```python
from build123d import *

# Parameters (mm, degrees)
SKETCH1_W           = 130
SKETCH1_H           = 79
BOSS_EXTRUDE1_DEPTH = 30
FILLET1_R           = 6
SHELL1_T            = -2.5
SKETCH2_W           = 130
SKETCH2_H           = 79
SKETCH2_W_2         = 127.5
SKETCH2_H_2         = 76.5
CUT_EXTRUDE1_DEPTH  = 3
SKETCH3_R           = 2
BOSS_EXTRUDE2_DEPTH = 8
BOSS_EXTRUDE3_REACH = 83.763
CUT_EXTRUDE2_REACH  = 108.611
SKETCH5_W           = 31.98
SKETCH5_H           = 7.98
SKETCH6_W           = 41.4
SKETCH6_H           = 24.3
CUT_EXTRUDE3_DEPTH  = 1.25
CUT_EXTRUDE4_REACH  = 108.611
SKETCH7_R           = 3.26


with BuildPart() as part:
    # Sketch1 → Boss-Extrude1 (new body)
    with BuildSketch(Plane(origin=(0, 0, 0), x_dir=(1, 0, 0), z_dir=(0, 1, 0))):
        Rectangle(SKETCH1_W, SKETCH1_H)
    extrude(amount=BOSS_EXTRUDE1_DEPTH)

    # Fillet1
    fillet1_edges = [part.edges().sort_by_distance(p)[0] for p in [
        (0, 0, 39.5),
        (-65, 0, 0),
        (0, 0, -39.5),
        (65, 0, 0),
    ]]
    fillet(fillet1_edges, radius=FILLET1_R)

    # Shell1
    shell1_openings = [part.faces().sort_by_distance(p)[0] for p in [
        (0, 30, 0),
    ]]
    offset(amount=SHELL1_T, openings=shell1_openings)

    # Sketch2 → Cut-Extrude1 (cut)
    with BuildSketch(Plane(origin=(0, 30, 0), x_dir=(1, 0, 0), z_dir=(0, 1, 0))):
        Rectangle(SKETCH2_W, SKETCH2_H)
        Rectangle(SKETCH2_W_2, SKETCH2_H_2, mode=Mode.SUBTRACT)
    extrude(amount=-CUT_EXTRUDE1_DEPTH, mode=Mode.SUBTRACT)

    # Sketch3 → Boss-Extrude2 (add)
    with BuildSketch(Plane(origin=(0, 2.5, 0), x_dir=(1, 0, 0), z_dir=(0, 1, 0))):
        with Locations(Location((-47.503765377, 21.122596556, 0), (0, 0, 90))):
            Circle(SKETCH3_R)
        with Locations(Location((33.776234623, 21.122596556, 0), (0, 0, 90))):
            Circle(SKETCH3_R)
        with Locations(Location((-47.503765377, -13.167403444, 0), (0, 0, 90))):
            Circle(SKETCH3_R)
        with Locations(Location((33.776234623, -13.167403444, 0), (0, 0, 90))):
            Circle(SKETCH3_R)
    extrude(amount=BOSS_EXTRUDE2_DEPTH)

    # Sketch4 → Boss-Extrude3 (add, up to next)
    with BuildSketch(Plane(origin=(0, 30, 0), x_dir=(1, 0, 0), z_dir=(0, 1, 0)), mode=Mode.PRIVATE) as boss_extrude3_sk1:
        with BuildLine():
            Line((-62.5, 37), (-62.5, 35.502936105))
            ThreePointArc((-62.5, 35.502936105), (-58.382233047, 32.882233047), (-61.002936105, 37))
            Line((-61.002936105, 37), (-62.5, 37))
        make_face()
    boss_extrude3_tool1 = extrude(boss_extrude3_sk1.sketch, amount=-BOSS_EXTRUDE3_REACH, mode=Mode.PRIVATE) - part.part
    # Sketch4 → Boss-Extrude3 (add, up to next)
    with BuildSketch(Plane(origin=(0, 30, 0), x_dir=(1, 0, 0), z_dir=(0, 1, 0)), mode=Mode.PRIVATE) as boss_extrude3_sk2:
        with BuildLine():
            Line((62.5, 37), (62.5, 35.502936105))
            ThreePointArc((62.5, 35.502936105), (58.382233047, 32.882233047), (61.002936105, 37))
            Line((61.002936105, 37), (62.5, 37))
        make_face()
    boss_extrude3_tool2 = extrude(boss_extrude3_sk2.sketch, amount=-BOSS_EXTRUDE3_REACH, mode=Mode.PRIVATE) - part.part
    # Sketch4 → Boss-Extrude3 (add, up to next)
    with BuildSketch(Plane(origin=(0, 30, 0), x_dir=(1, 0, 0), z_dir=(0, 1, 0)), mode=Mode.PRIVATE) as boss_extrude3_sk3:
        with BuildLine():
            Line((-62.5, -37), (-62.5, -35.502936105))
            ThreePointArc((-62.5, -35.502936105), (-58.382233047, -32.882233047), (-61.002936105, -37))
            Line((-61.002936105, -37), (-62.5, -37))
        make_face()
    boss_extrude3_tool3 = extrude(boss_extrude3_sk3.sketch, amount=-BOSS_EXTRUDE3_REACH, mode=Mode.PRIVATE) - part.part
    # Sketch4 → Boss-Extrude3 (add, up to next)
    with BuildSketch(Plane(origin=(0, 30, 0), x_dir=(1, 0, 0), z_dir=(0, 1, 0)), mode=Mode.PRIVATE) as boss_extrude3_sk4:
        with BuildLine():
            Line((62.5, -37), (61.002936105, -37))
            ThreePointArc((61.002936105, -37), (58.382233047, -32.882233047), (62.5, -35.502936105))
            Line((62.5, -35.502936105), (62.5, -37))
        make_face()
    boss_extrude3_tool4 = extrude(boss_extrude3_sk4.sketch, amount=-BOSS_EXTRUDE3_REACH, mode=Mode.PRIVATE) - part.part
    add(boss_extrude3_tool1.solids().sort_by_distance((-60.224191, 30, -34.724191))[0])
    add(boss_extrude3_tool2.solids().sort_by_distance((60.224191, 30, -34.724191))[0])
    add(boss_extrude3_tool3.solids().sort_by_distance((-60.224191, 30, 34.724191))[0])
    add(boss_extrude3_tool4.solids().sort_by_distance((60.224191, 30, 34.724191))[0])

    # Cut-Extrude2: up to this face of the body (flat: up to its plane)
    cut_extrude2_end = Plane(part.part.faces().sort_by_distance((0, 18, 37))[0])
    # Sketch5 → Cut-Extrude2 (cut, up to the picked face)
    with BuildSketch(Plane.XY.offset(39.5), mode=Mode.PRIVATE) as cut_extrude2_sk1:
        with Locations((0, 26.01)):
            Rectangle(SKETCH5_W, SKETCH5_H)
    cut_extrude2_tool1 = split(extrude(cut_extrude2_sk1.sketch, amount=-CUT_EXTRUDE2_REACH, mode=Mode.PRIVATE), bisect_by=cut_extrude2_end, keep=Keep.BOTH, mode=Mode.PRIVATE)
    add(cut_extrude2_tool1.solids().sort_by(Axis((0, 26.01, 39.5), (0, 0, -1)))[0], mode=Mode.SUBTRACT)

    # Sketch6 → Cut-Extrude3 (cut)
    with BuildSketch(Plane(origin=(0, 0, 37), x_dir=(-1, 0, 0), z_dir=(0, 0, -1))):
        with Locations((0, 22.66)):
            Rectangle(SKETCH6_W, SKETCH6_H)
    extrude(amount=-CUT_EXTRUDE3_DEPTH, mode=Mode.SUBTRACT)

    # Sketch7 → Cut-Extrude4 (cut, up to next)
    with BuildSketch(Plane.XY.offset(39.5), mode=Mode.PRIVATE) as cut_extrude4_sk1:
        with Locations((-40.495, 20)):
            Circle(SKETCH7_R)
    cut_extrude4_tool1 = extrude(cut_extrude4_sk1.sketch, amount=-CUT_EXTRUDE4_REACH, mode=Mode.PRIVATE) & part.part
    add(cut_extrude4_tool1.solids().sort_by_distance((-40.495, 20, 39.5))[0], mode=Mode.SUBTRACT)


solid = part.part
```
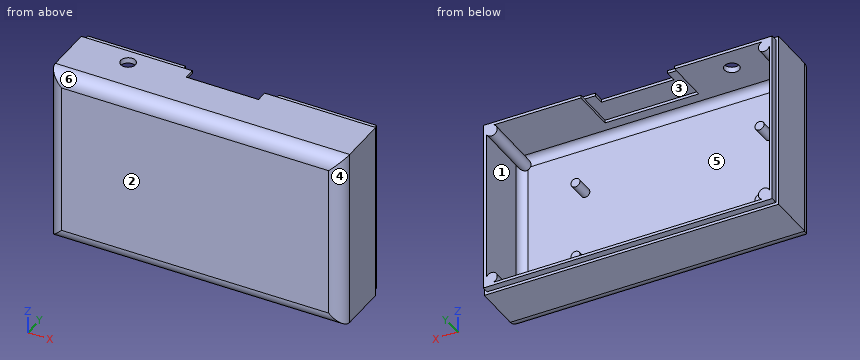
Geometry: final body of the model. Coordinates: model frame, mm. Face numbers are marked on the shaded views. A direction names the side the tool comes from. Give positions to 0.01 mm unless a question says otherwise; leave off trailing zeros. Loops run counter-clockwise (first coordinate to the right, second up) from the corner with the lowest first, then second, coordinate; pieces in that order, holes last. Notation, with made-up numbers: (-38.5, 33.25) - (-34.5, 33.25) arc R7 cw to (-34.5, 37.25) - close; hole circle Ø1 at (18, 88). An arc over 180 degrees is marked (long way). Answer as CSV lines item,"result". Start each with the question number.
(1) Pin query (flat end, axial travel): P1, Ø1.5, axis at x = -42, y = 28, coming from the +Z side; P2, Ø2, axis at x = 33.5, z = -22, coming from the +Y side; P3, Ø23.5, axis at x = 9.5, z = -19.5, coming from the +Y side. Return the tip coordinate at first contact, or that it passes through.
(2) Mould query, pull axis X, two halves, no side actions, for the marked faces 1, 2, 3 and 4. Classes: +X half, -X half, draft (parallel to the pull), parting line (faces both ways), or undercut.
(3) Ray query, line 1 along X through (y, z) = (18, -18); line 2 along Z through (x, y) = (-10, 14); line 3 along Z through (x, y) = (34, 21.5). Return the intervals inside material, ascending. Write a range as [from, to].
(4) Section query B-B (x = -3). Output: boundary loops of the cut face in (y, z), and give its area (3 significant figures).
(5) Section query A-A (z = -13). Output: boundary loops of the cut face in (x, y).
(6) Section query C-C (z = -21). Output: boundary loops of the cut face in (x, y).
(7) Reachability of the marked faces 5 and 6 from +Z, -Z, +X, -X, +Y, -Y: full face, straight path, thin tool, end or side. Return the list, or none.
Worked answers:
1,P1,"stops at z = 38.25"
1,P2,"stops at y = 10.5"
1,P3,"stops at y = 2.5"
2,face 1,"undercut"
2,face 2,"draft"
2,face 3,"undercut"
2,face 4,"+X half"
3,line 1,"x = [-65, -62.5], [62.5, 65]"
3,line 2,"z = [-39.5, -37], [38.25, 39.5]"
3,line 3,"z = [-39.5, -37], [37, 39.5]"
4,outline,"(0, -33.5) arc R6 ccw to (6, -39.5) - (27, -39.5) - (27, -38.25) - (30, -38.25) - (30, -37) - (6, -37) arc R3.5 cw to (2.5, -33.5) - (2.5, 33.5) arc R3.5 cw to (6, 37) - (10.51, 37) - (10.51, 38.25) - (22.02, 38.25) - (22.02, 39.5) - (6, 39.5) arc R6 ccw to (0, 33.5) - close"
4,area,"287 mm^2"
5,outline,"(-65, 6) arc R6 ccw to (-59, 0) - (59, 0) arc R6 ccw to (65, 6) - (65, 27) - (63.75, 27) - (63.75, 30) - (62.5, 30) - (62.5, 6) arc R3.5 cw to (59, 2.5) - (-59, 2.5) arc R3.5 cw to (-62.5, 6) - (-62.5, 30) - (-63.75, 30) - (-63.75, 27) - (-65, 27) - close"
6,outline,"(-65, 6) arc R6 ccw to (-59, 0) - (59, 0) arc R6 ccw to (65, 6) - (65, 27) - (63.75, 27) - (63.75, 30) - (62.5, 30) - (62.5, 6) arc R3.5 cw to (59, 2.5) - (35.77, 2.5) - (35.77, 10.5) - (31.78, 10.5) - (31.78, 2.5) - (-45.51, 2.5) - (-45.51, 10.5) - (-49.5, 10.5) - (-49.5, 2.5) - (-59, 2.5) arc R3.5 cw to (-62.5, 6) - (-62.5, 30) - (-63.75, 30) - (-63.75, 27) - (-65, 27) - close"
7,face 5,"+Y"
7,face 6,"+Z, +X, -X, -Y"
